Read the model definition and answer for the solid it produces. Units are mm, in the model's axes. Give positions to 0.01 mm unless a question says otherwise; leave off trailing zeros. Write each loop counter-clockwise with the first axis right and the second up, starting at its lowest first coordinate (ties: lowest second). Pieces come first, ordered by that corner, then holes. Notation, with made-up numbers: M -36,13 L 16,13 A22 ccw 16,25 Z; hole C 10.25,-39 d11. An arc over 180 degrees is marked long. Use a Markdown table: item, result. Add a question column.
Item 1: Given P1, Ø0.9, axis at x = -41.5, y = -1, coming from the +Z side; P2, Ø0.9, axis at y = -2, z = -40.5, coming from the -X side; P3, Ø2.5, axis at y = -1, z = -42, coming from the +X side, each flat-ended and moving along its own axis, determine where each tip first touches the part or whether it passes through.
Item 2: A cutting plane is placed at C-C on z = 35. Determine the outline of the cut face in (x, y), then the cut area to 3 significant figures.
Item 3: A cutting plane is placed at B-B on z = 0. Determine the outline of the cut face in (x, y).
Item 4: A cutting plane is placed at A-A on x = 0. Determine the outline of the cut face in (y, z).
Item 5: A cutting plane is placed at D-D on y = 1.5. Determine the outline of the cut face in (x, z), then the cut area to 3 significant figures.
Item 6: Consider probe 1 along X at (y, z) = (1.5, 0); probe 2 along X at (y, z) = (-2, 49); probe 3 along X at (y, z) = (-2.5, -44). Determine where each line is inside the solid, lowest interval first. Write a range as [from, to].
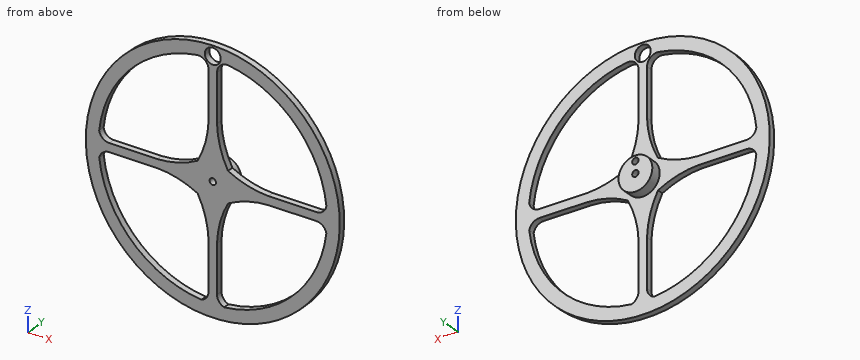
from build123d import *

# Parameters (mm, degrees)
SKETCH1_R           = 60
SKETCH1_R_2         = 54
SKETCH1_R_3         = 8
BOSS_EXTRUDE1_DEPTH = 3
SKETCH1_3_R         = 8
BOSS_EXTRUDE2_DEPTH = 5
CUT_EXTRUDE1_REACH  = 87.229
SKETCH2_R           = 1.5
CUT_EXTRUDE2_REACH  = 87
SKETCH3_R           = 3.75
SKETCH4_R           = 1.5
CUT_EXTRUDE3_DEPTH  = 5


with BuildPart() as part:
    # Sketch1 → Boss-Extrude1 (new body)
    # profile 1 of 3: a face of its own
    with BuildSketch(Plane(origin=(0, 0, 0), x_dir=(1, 0, 0), z_dir=(0, 1, 0))):
        with Locations(Location((0, 0, 0), (0, 0, 270))):
            Circle(SKETCH1_R)
        Circle(SKETCH1_R_2, mode=Mode.SUBTRACT)
    # profile 2 of 3: a face of its own
    with BuildSketch(Plane(origin=(0, 0, 0), x_dir=(1, 0, 0), z_dir=(0, 1, 0))):
        with BuildLine():
            ThreePointArc((7.5, -53.47663041), (3.660460389, -52.338407931), (2.000000204, -48.694167705))
            Line((2.000000204, -48.694167705), (2.000000204, -26.109482291))
            ThreePointArc((2.000000204, -26.109482291), (3.464837403, -16.231345149), (7.178910038, -6.961555191))
            ThreePointArc((7.178910038, -6.961555191), (16.451417639, -3.257530466), (26.326837138, -1.782645358))
            Line((26.326837138, -1.782645358), (48.911522552, -1.782645358))
            ThreePointArc((48.911522552, -1.782645358), (52.048100377, -2.939896306), (53.681424467, -5.857018624))
            ThreePointArc((53.681424467, -5.857018624), (53.920297297, -2.93283811), (54, 0))
            ThreePointArc((54, 0), (53.912855321, 3.066599276), (53.651702551, 6.123300855))
            ThreePointArc((53.651702551, 6.123300855), (51.982585847, 3.31964037), (48.911522552, 2.217355051))
            Line((48.911522552, 2.217355051), (26.326837138, 2.217355051))
            ThreePointArc((26.326837138, 2.217355051), (16.448699996, 3.682192249), (7.178910038, 7.396264884))
            ThreePointArc((7.178910038, 7.396264884), (3.474885313, 16.668772485), (2.000000204, 26.544191985))
            Line((2.000000204, 26.544191985), (2.000000204, 49.128877399))
            ThreePointArc((2.000000204, 49.128877399), (2.932488129, 51.981408674), (5.369841962, 53.732344052))
            ThreePointArc((5.369841962, 53.732344052), (0, 54), (-5.369841962, 53.732344052))
            ThreePointArc((-5.369841962, 53.732344052), (-2.932488129, 51.981408674), (-2.000000204, 49.128877399))
            Line((-2.000000204, 49.128877399), (-2.000000204, 26.544191985))
            ThreePointArc((-2.000000204, 26.544191985), (-3.464837403, 16.666054843), (-7.178910038, 7.396264884))
            ThreePointArc((-7.178910038, 7.396264884), (-16.451417639, 3.69224016), (-26.326837138, 2.217355051))
            Line((-26.326837138, 2.217355051), (-48.911522552, 2.217355051))
            ThreePointArc((-48.911522552, 2.217355051), (-51.982585847, 3.31964037), (-53.651702551, 6.123300855))
            ThreePointArc((-53.651702551, 6.123300855), (-53.99983382, 0.133967924), (-53.681424467, -5.857018624))
            ThreePointArc((-53.681424467, -5.857018624), (-52.048100377, -2.939896306), (-48.911522552, -1.782645358))
            Line((-48.911522552, -1.782645358), (-26.326837138, -1.782645358))
            ThreePointArc((-26.326837138, -1.782645358), (-16.448699996, -3.247482556), (-7.178910038, -6.961555191))
            ThreePointArc((-7.178910038, -6.961555191), (-3.474885313, -16.234062792), (-2.000000204, -26.109482291))
            Line((-2.000000204, -26.109482291), (-2.000000204, -48.694167705))
            ThreePointArc((-2.000000204, -48.694167705), (-3.660460389, -52.338407931), (-7.5, -53.47663041))
            ThreePointArc((-7.5, -53.47663041), (0, -54), (7.5, -53.47663041))
        make_face()
        Circle(SKETCH1_R_3, mode=Mode.SUBTRACT)
    # profile 3 of 3: a face of its own
    with BuildSketch(Plane(origin=(0, 0, 0), x_dir=(1, 0, 0), z_dir=(0, 1, 0))):
        Circle(SKETCH1_R_3)
    extrude(amount=-BOSS_EXTRUDE1_DEPTH)

    # Sketch1<3> → Boss-Extrude2 (add)
    with BuildSketch(Plane(origin=(0, 0, 0), x_dir=(1, 0, 0), z_dir=(0, 1, 0))):
        with Locations(Location((0, 0, 0), (0, 0, 270))):
            Circle(SKETCH1_3_R)
    extrude(amount=BOSS_EXTRUDE2_DEPTH)

    # Sketch2 → Cut-Extrude1 (cut, up to next)
    with BuildSketch(Plane(origin=(0, 5, 0), x_dir=(1, 0, 0), z_dir=(0, 1, 0)), mode=Mode.PRIVATE) as cut_extrude1_sk1:
        with Locations(Location((0, 0, 0), (0, 0, 270))):
            Circle(SKETCH2_R)
    cut_extrude1_tool1 = extrude(cut_extrude1_sk1.sketch, amount=-CUT_EXTRUDE1_REACH, mode=Mode.PRIVATE) & part.part
    add(cut_extrude1_tool1.solids().sort_by_distance((0, 5, 0))[0], mode=Mode.SUBTRACT)

    # Sketch3 → Cut-Extrude2 (cut, up to next)
    with BuildSketch(Plane(origin=(0, 0, 0), x_dir=(1, 0, 0), z_dir=(0, 1, 0)), mode=Mode.PRIVATE) as cut_extrude2_sk1:
        with Locations(Location((0, -55.25, 0), (0, 0, 270))):
            Circle(SKETCH3_R)
    cut_extrude2_tool1 = extrude(cut_extrude2_sk1.sketch, amount=-CUT_EXTRUDE2_REACH, mode=Mode.PRIVATE) & part.part
    add(cut_extrude2_tool1.solids().sort_by_distance((0, 0, 55.25))[0], mode=Mode.SUBTRACT)

    # Sketch4 → Cut-Extrude3 (cut)
    with BuildSketch(Plane(origin=(0, 5, 0), x_dir=(1, 0, 0), z_dir=(0, 1, 0))):
        with Locations(Location((0, -5.5, 0), (0, 0, 270))):
            Circle(SKETCH4_R)
    extrude(amount=-CUT_EXTRUDE3_DEPTH, mode=Mode.SUBTRACT)


solid = part.part
Filled in:
| question | item | result |
|---|---|---|
| 1 | P1 | z = 43.76 |
| 1 | P2 | x = -44.68 |
| 1 | P3 | x = 44.04 |
| 2 | outline | M -48.73,-3 L -41.12,-3 L -41.12,0 L -48.73,0 Z; M -2,-3 L 2,-3 L 2,0 L -2,0 Z; M 41.12,-3 L 48.73,-3 L 48.73,0 L 41.12,0 Z |
| 2 | area | 57.7 mm² |
| 3 | outline | M -60,-3 L -1.5,-3 L -1.5,5 L -8,5 L -8,0 L -60,0 Z; M 1.5,-3 L 60,-3 L 60,0 L 8,0 L 8,5 L 1.5,5 Z |
| 4 | outline | M -3,-60 L 0,-60 L 0,-8 L 5,-8 L 5,-1.5 L -3,-1.5 Z; M -3,1.5 L 5,1.5 L 5,4 L 0,4 L 0,7 L 5,7 L 5,8 L 0,8 L 0,51.5 L -3,51.5 Z; M -3,59 L 0,59 L 0,60 L -3,60 Z |
| 5 | outline | C 0,0 d16; hole C 0,0 d3; hole C 0,5.5 d3 |
| 5 | area | 187 mm² |
| 6 | probe 1 | [-8, -1.5], [1.5, 8] |
| 6 | probe 2 | [-34.63, -22.69], [-2.01, 2.01], [22.69, 34.63] |
| 6 | probe 3 | [-40.79, -31.3], [-2, 2], [31.3, 40.79] |
